```python
from build123d import *

# Parameters (mm, degrees)
SKETCH1_R                = 34.925
EXTRUDE1_DEPTH           = 12.7
SKETCH2_R                = 4.7625
CUT_EXTRUDE1_DEPTH       = 51.998051433
SKETCH3_R                = 3.3655
CUT_EXTRUDE2_DEPTH       = 51.998051433
CIRPATTERN1_COUNT        = 6
EXTRUDE_THIN1_DEPTH      = 45.72
EXTRUDE_THIN1_DEPTH_BACK = 17.78
SKETCH5_R                = 4.7625
SKETCH5_R_2              = 4.1275


with BuildPart() as part:
    # Sketch1 → Extrude1 (new body)
    with BuildSketch(Plane(origin=(0, 0, 0), x_dir=(1, 0, 0), z_dir=(0, 1, 0))):
        with Locations(Location((0, 0, 0), (0, 0, 270))):
            Circle(SKETCH1_R)
    extrude(amount=EXTRUDE1_DEPTH)

    # Sketch2 → Cut-Extrude1 (cut, through all)
    with BuildSketch(Plane(origin=(0, 0, 0), x_dir=(1, 0, 0), z_dir=(0, 1, 0))):
        with Locations(Location((0, 0, 0), (0, 0, 270))):
            Circle(SKETCH2_R)
    extrude(amount=CUT_EXTRUDE1_DEPTH, mode=Mode.SUBTRACT)

    # Sketch3 → Cut-Extrude2 (cut, through all)
    with BuildSketch(Plane(origin=(0, 0, 0), x_dir=(1, 0, 0), z_dir=(0, 1, 0))):
        with Locations(Location((0, 29.337, 0), (0, 0, 270))):
            Circle(SKETCH3_R)
    cut_extrude2 = extrude(amount=CUT_EXTRUDE2_DEPTH, mode=Mode.SUBTRACT)

    # CirPattern1: Cut-Extrude2 ×6 about axis
    cirpattern1_axis = Axis((0, 0, 0), (0, 1, 0))
    for i in range(1, CIRPATTERN1_COUNT):
        add(cut_extrude2.rotate(cirpattern1_axis, i * 360 / CIRPATTERN1_COUNT), mode=Mode.SUBTRACT)

    # Sketch5 → Extrude-Thin1 (add, two sides: drawn at the far end of the back side and taken through both)
    with BuildSketch(Plane.XZ.offset(-EXTRUDE_THIN1_DEPTH_BACK)):
        Circle(SKETCH5_R)
        Circle(SKETCH5_R_2, mode=Mode.SUBTRACT)
    extrude(amount=EXTRUDE_THIN1_DEPTH + EXTRUDE_THIN1_DEPTH_BACK)


solid = part.part
```
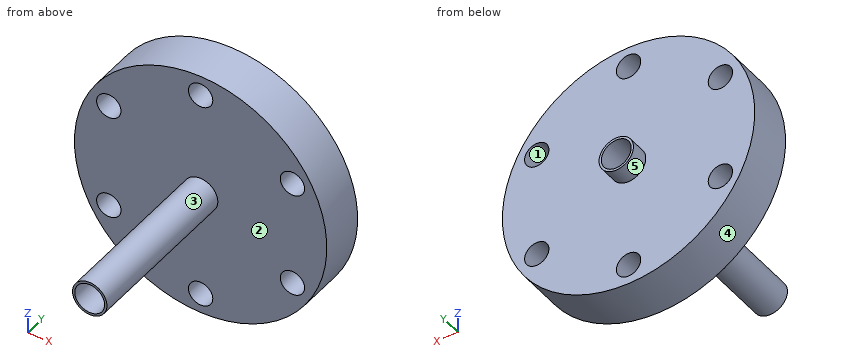
Design review of the part built by this model. Coordinates are the model's own, in mm. Face numbers are marked on the shaded views. A direction names the side the tool comes from. Give positions to 0.01 mm unless a question says otherwise; leave off trailing zeros. Order: outer loops, then holes, each group sorted by start corner. A loop starts at its lowest first (then second) coordinate and runs counter-clockwise, first axis right, second up. Notation, with made-up numbers: (-39, 1.25) -> (17, 1.25) arc R20 cw to (17, 6.25) -> close; hole circle Ø5 at (0, 85). An arc over 180 degrees is marked (long way). Write item = value, one per line. Start each with the question number.
(1) To check wall thickness, follow line 1 along Z through (x, y) = (-1, 2); line 2 along Y through (x, z) = (-25, -6); line 3 along Z through (x, y) = (1, -24.5). State the ranges of each line that lie inside material, in increasing order.
(2) For pin 1 (5 mm diameter, centred on y = -25, z = -2.5, fed in from +X); pin 2 (6 mm diameter, centred on y = 11, z = 26, fed in from +X); pin 3 (8 mm diameter, centred on x = -19.5, z = 14, fed in from +Y), all flat-tipped, find the tip position at first contact; note any pin that passes through.
(3) We need section C-C on y = -7. Write out the cut boundary in (x, z) (1 decimal).
(4) For the marked faces 4 and 5, list the 3-axis set-ups (+Z, -Z, +X, -X, +Y, -Y) from which the entire face can be reached by the end or side of a thin tool; tool diameter is ignored.
(5) We need section B-B on z = 0. Write out the cut boundary in (x, y) (1 decimal), plus the area to 3 significant figures.
(6) Mouldability with a two-part tool opening along Z and no side actions: class the marked faces 1, 2 and 3 as +Z half, -Z half, draft (parallel to the pull), parting line (faces both ways), or undercut.
(7) We need section A-A on x = 0. Write out the cut boundary in (y, z) (1 decimal), plus the area to 3 significant figures.
(8) We need section D-D on x = -23.5. Write out the cut boundary in (y, z), plus the area to 3 significant figures.
Numbers:
q1.line_1 = -34.91 to -32.55, -26.12 to -4, 4 to 26.12, 32.55 to 34.91
q1.line_2 = 0 to 12.7
q1.line_3 = -4.66 to -4, 4 to 4.66
q2.pin_1 = 4.76
q2.pin_2 = 26.28
q2.pin_3 = 12.7
q3.outline = circle Ø9.5 at (0, 0); hole circle Ø8.3 at (0, 0)
q4.face_4 = +Y, -Y
q4.face_5 = +Y
q5.outline = (-34.9, 0) -> (-4.8, 0) -> (-4.8, -45.7) -> (-4.1, -45.7) -> (-4.1, 17.8) -> (-4.8, 17.8) -> (-4.8, 12.7) -> (-34.9, 12.7) -> close; (4.1, -45.7) -> (4.8, -45.7) -> (4.8, 0) -> (34.9, 0) -> (34.9, 12.7) -> (4.8, 12.7) -> (4.8, 17.8) -> (4.1, 17.8) -> close
q5.area = 847 mm^2
q6.face_1 = undercut
q6.face_2 = draft
q6.face_3 = parting line
q7.outline = (-45.7, -4.8) -> (0, -4.8) -> (0, -26) -> (12.7, -26) -> (12.7, -4.8) -> (17.8, -4.8) -> (17.8, -4.1) -> (-45.7, -4.1) -> close; (-45.7, 4.1) -> (17.8, 4.1) -> (17.8, 4.8) -> (12.7, 4.8) -> (12.7, 26) -> (0, 26) -> (0, 4.8) -> (-45.7, 4.8) -> close; (0, -34.9) -> (12.7, -34.9) -> (12.7, -32.7) -> (0, -32.7) -> close; (0, 32.7) -> (12.7, 32.7) -> (12.7, 34.9) -> (0, 34.9) -> close
q7.area = 676 mm^2
q8.outline = (0, -25.84) -> (12.7, -25.84) -> (12.7, -17.44) -> (0, -17.44) -> close; (0, -11.9) -> (12.7, -11.9) -> (12.7, 11.9) -> (0, 11.9) -> close; (0, 17.44) -> (12.7, 17.44) -> (12.7, 25.84) -> (0, 25.84) -> close
q8.area = 515 mm^2
